Can you work these out from the model? Positions are in its coordinate system, mm. A direction names the side the tool comes from. Round coordinates to 2 decimals unless told otherwise and drop trailing zeros. Order: outer loops, then holes, each group sorted by start corner. A loop starts at its lowest first (then second) coordinate and runs counter-clockwise, first axis right, second up. Notation, with made-up numbers: M 56,-4 L 102,-4 A22 ccw 102,7 Z; hole C -22.5,54 d9. An arc over 180 degrees is marked long. One line per question, with ' | ' between items.
```python
from build123d import *

# Parameters (mm, degrees)
SKETCH1_W               = 15
SKETCH1_H               = 7.5
BOSS_EXTRUDE1_DEPTH     = 6
SKETCH2_R               = 1.25
CUT_EXTRUDE1_DEPTH      = 6
FILLET1_R               = 3.75
CUT_EXTRUDE2_DEPTH      = 23.639843197
CUT_EXTRUDE2_DEPTH_BACK = 23.639843197
SKETCH3_W               = 5
SKETCH3_H               = 3
FILLET2_R               = 2


with BuildPart() as part:
    # Sketch1 → Boss-Extrude1 (new body)
    with BuildSketch(Plane(origin=(0, 0, 0), x_dir=(1, 0, 0), z_dir=(0, 1, 0))):
        Polygon((-20, 3.75), (-12.5, 3.75), (-12.5, 8.75), (12.5, 8.75), (12.5, 3.75), (20, 3.75), (20, -3.75), (12.5, -3.75), (12.5, -8.75), (-12.5, -8.75), (-12.5, -3.75), (-20, -3.75), align=None)
        Rectangle(SKETCH1_W, SKETCH1_H, mode=Mode.SUBTRACT)
    extrude(amount=BOSS_EXTRUDE1_DEPTH)

    # Sketch2 → Cut-Extrude1 (cut)
    with BuildSketch(Plane(origin=(0, 0, 0), x_dir=(1, 0, 0), z_dir=(0, 1, 0))):
        with Locations(Location((-10.75, 0, 0), (0, 0, 270))):
            Circle(SKETCH2_R)
        with Locations(Location((10.75, 0, 0), (0, 0, 90))):
            Circle(SKETCH2_R)
    extrude(amount=CUT_EXTRUDE1_DEPTH, mode=Mode.SUBTRACT)

    # Fillet1
    fillet1_edges = [part.edges().sort_by_distance(p)[0] for p in [
        (-20, 3, 3.75),
        (-20, 3, -3.75),
        (20, 3, 3.75),
        (20, 3, -3.75),
    ]]
    fillet(fillet1_edges, radius=FILLET1_R - 0.0001)  # a hair under: the kernel refuses the full size

    # Sketch3 → Cut-Extrude2 (cut, two sides: drawn at the far end of the back side and taken through both)
    with BuildSketch(Plane(origin=(0, 0, 0), x_dir=(0, 0, -1), z_dir=(1, 0, 0)).offset(-CUT_EXTRUDE2_DEPTH_BACK)):
        with Locations((6.25, 4.5)):
            Rectangle(SKETCH3_W, SKETCH3_H)
        with Locations((-6.25, 4.5)):
            Rectangle(SKETCH3_W, SKETCH3_H)
    extrude(amount=CUT_EXTRUDE2_DEPTH + CUT_EXTRUDE2_DEPTH_BACK, mode=Mode.SUBTRACT)

    # Fillet2
    fillet2_edges = [part.edges().sort_by_distance(p)[0] for p in [
        (12.5, 1.5, 3.75),
        (12.5, 1.5, 8.75),
        (-12.5, 1.5, 8.75),
        (-12.5, 1.5, 3.75),
        (-12.5, 1.5, -3.75),
        (-12.5, 1.5, -8.75),
        (12.5, 1.5, -8.75),
        (12.5, 1.5, -3.75),
    ]]
    fillet(fillet2_edges, radius=FILLET2_R)


solid = part.part
```
(1) If we section it at D-D on z = -2.25: Please give me the cut outline in (x, y), plus the area to 3 significant figures.
Final values:
outline: M -19.25,0 L -7.5,0 L -7.5,6 L -19.25,6 Z; M 7.5,0 L 19.25,0 L 19.25,6 L 7.5,6 Z | area: 141 mm^2
(2) If we section it at C-C on x = -8: Please give me the cut outline in (y, z), plus the area to 3 significant figures.
Final values:
outline: M 0,-8.75 L 3,-8.75 L 3,-3.75 L 6,-3.75 L 6,3.75 L 3,3.75 L 3,8.75 L 0,8.75 Z | area: 75.0 mm^2
(3) Will these pins go through, and if not, where does the flat tip stop? pin 1 Ø0.5 at (y, z) = (2, 6) entering from -X; pin 2 Ø1.1 at (y, z) = (1.5, -6.5) entering from +X; pin 3 Ø4 at (x, z) = (-4.5, -6) entering from +Y.
Final values:
pin 1: x = -12.5 | pin 2: x = 12.5 | pin 3: y = 3
(4) On a 3-axis mill with a long thin cutter (end or side, diameter ignored), from which of +Z, -Z, +X, -X, +Y, -Y can I reach the whole of each face in a straight line? I mean faces 1 (the flat face through (13, 4, -3.75)), 2 (the flat face through (-12.5, 1, -6)), 3 (the flat face through (0, 1, 3.75)), 4 (the flat face through (12.5, 1, -6)), 5 (the flat face through (0, 3, 6)). Say none if no direction works.
Final values:
face 1: -Z, +X, +Y | face 2: -Z, -X, +Y, -Y | face 3: +Y, -Y | face 4: -Z, +X, +Y, -Y | face 5: +Z, +X, -X, +Y
(5) Please list where these lines run through material, in increasing order: probe 1 along X at (y, z) = (3.35, 0); probe 2 along X at (y, z) = (0.3, -0.5); probe 3 along Z at (x, y) = (10.75, 3.3). Write a range as [from, to].
Final values:
probe 1: [-20, -12], [-9.5, -7.5], [7.5, 9.5], [12, 20] | probe 2: [-19.97, -11.9], [-9.6, -7.5], [7.5, 9.6], [11.9, 19.97] | probe 3: [-3.75, -1.25], [1.25, 3.75]
(6) If we section it at A-A on y = 3.8: State how many separate pieces and enclosed holes the cut face has, plus the area to 3 significant figures.
Final values:
separate pieces: 2 | enclosed holes: 2 | area: 166 mm^2
(7) If we section it at B-B on x = 1: Please give me the cut outline in (y, z).
Final values:
outline: M 0,-8.75 L 3,-8.75 L 3,-3.75 L 0,-3.75 Z; M 0,3.75 L 3,3.75 L 3,8.75 L 0,8.75 Z
